Autodesk Inventor part; units mm, degrees
ref_plane "Work Plane1" through (29, 0, 0) normal (0, -1, 0) x (1, 0, 0)
ref_plane "YZ Plane" through (0, 0, 0) normal (1, 0, 0) x (0, 1, 0)
ref_plane "XZ Plane" through (0, 0, 0) normal (0, 1, 0) x (-1, 0, 0)
sketch "Эскиз1" plane through (0, 0, 0) normal (0, 0, 1) x (1, 0, 0)
  line L0 (-1, 0) -> (6, 0)
  line L1 (6, 0) -> (6, 2)
  line L2 (6, 2) -> (2.1, 2)
  line L3 (2.1, 2) -> (1.6705, 2)
  line L4 (1.6705, 2) -> (0, 2)
  line L5 (0, 2) -> (0, 3.5)
  line L6 (0, 3.5) -> (-4, 3.5)
  line L7 (-4, 3.5) -> (-4, 1.7321)
  line L8 (-4, 1.7321) -> (-2, 1.7321)
  line L9 (-2, 1.7321) -> (-1, 0)
  line L10 (-6, 0) -> (8, 0)
  line L11 (0, -0.7) -> (0, 4.2)
  line L12 (2.1, 2) -> (0, 2) construction
  dimension "d1" = 3.9
  dimension "d2" = 0.4295
  dimension "d3" = 4
  dimension "d4" = 2
  dimension "d5" = 60
  dimension "d6" = 4
  dimension "d7" = 4
  dimension "d8" = 3.4641
  dimension "d9" = 7
  dimension "d26" = 6
revolve "Базовый элемент" add sketch "Эскиз1" angle 360 about axis through (-1, 0, 0) along (1, 0, 0)
sketch "Эскиз2" plane through (-4, 0, 0) normal (-1, 0, 0) x (0, 0, 1)
  circle A0 centre (0, 0) radius 1.7321
  line L0 (0, -4.9) -> (0, 4.9)
  line L1 (-4.9, 0) -> (4.9, 0)
  line L2 (1.7321, 0) -> (0.866, -1.5)
  line L3 (0.866, -1.5) -> (-0.866, -1.5)
  line L4 (-0.866, -1.5) -> (-1.7321, 0)
  line L5 (-1.7321, 0) -> (-0.866, 1.5)
  line L6 (-0.866, 1.5) -> (0.866, 1.5)
  line L7 (0.866, 1.5) -> (1.7321, 0)
extrude "Паз" add sketch "Эскиз2" against normal up to next contours L7 A0 | A0 L2 | L6 L0 A0 | A0 L0 L3 | L0 L6 A0 | A0 L3 L0 | L4 A0 | A0 L5
fillet "Сопряжение1" radius 0.4 1 edges at (-4, -3.5, 0)
thread "Резьба"
chamfer "Фаска1" distance 0.4294 distance2 0.4294 1 edges at (6, -2, 0) measured on face at (6, 0.556, 0.0273)
ref_plane "Work Plane1" through (29, 0, 0) normal (0, -1, 0) x (1, 0, 0)
fillet "Fillet2" radius 0.1 1 edges at (0, -2, 0)
equation "\"d1\" = GEL"
equation "\"d3\" = KOH"
equation "\"d4\" = INTI"
equation "\"d6\" = GD"
equation "\"d7\" = BDM"
equation "\"d8\" = 1.1547 * SW"
equation "\"d9\" = KOD"
equation "\"d26\" = NLG"
equation "\"d30\" = R"
equation "\"d17\" = RR"
equation "\"d13\" = GEL"
equation "\"d15\" = -0.5 * SPD + 0.5 * GD"
equation "\"d16\" = GUL"
equation "\"GD\" = NND"
equation "\"NLG\" = 6"
equation "\"GEL\" = 3.9"
equation "\"KOD\" = 7"
equation "\"KOH\" = NND"
equation "\"INTI\" = 2"
equation "\"GAL\" = 0.61345 * PTC"
equation "\"GUL\" = 0.61345 * PTC"
equation "\"BDM\" = NND"
equation "\"SW\" = 3"
equation "\"RR\" = 0.4"
equation "\"SPD\" = NND - 1.2269 * PTC"
equation "\"R\" = 0.1"
equation "\"TOA\" = 30deg"
equation "\"GD1\" = THREADDIA - 1.2269 * PTC"
equation "\"THREADDIA\" = 4"
equation "\"FAWI\" = 45deg"
equation "\"PTC\" = 0.7"
equation "\"NND\" = 4"
equation "\"E0\" = 1.155 * SW"
equation "\"PHH\" = 0"
properties part number "CSN 02 1143 - M4 x 6" material "Сталь, мягкая"
Design review of the part built by this model. Coordinates are the model's own, in mm. A direction names the side the tool comes from. Coordinates: 2 decimals unless noted, no trailing zeros. Order: outer loops, then holes, each group sorted by start corner. A loop starts at its lowest first (then second) coordinate and runs counter-clockwise, first axis right, second up. Notation, with made-up numbers: M -32,28.5 L -27,28.5 A24 ccw -27,55.5 Z; hole C -7,14 d4. An arc over 180 degrees is marked long. Use a Markdown table: item, result.
(1) Draft analysis for pull direction Z (two halves, no side actions). For faces 3 (the cylindrical face through (3, 0, 2)), 4 (the flat face through (0, 2, -2)), 5 (the flat face through (-3, 1.5, 0)), 6 (the flat face through (-2.948, 0.761, 1.293)), state which applies: released by +Z, released by -Z, zero draft, split by the parting line, or undercut.
Worked answers:
| item | result |
|---|---|
| face 3 | split by the parting line |
| face 4 | zero draft |
| face 5 | undercut |
| face 6 | undercut |
(2) Wall thickness on probe 1 along X at (y, z) = (0, 2.5); probe 2 along Z at (x, y) = (3.25, -1); probe 3 along Z at (x, y) = (-2.25, -1): over which ranges is each line inside the solid? List them lowest first.
Worked answers:
| item | result |
|---|---|
| probe 1 | x = -4 to 0 |
| probe 2 | z = -1.73 to 1.73 |
| probe 3 | z = -3.35 to -1.15, 1.15 to 3.35 |
(3) Add section A-A (x = -3). Give the boundary of the cut face in (y, z), then the cut area to 3 significant figures.
Worked answers:
| item | result |
|---|---|
| outline | C 0,0 d7; hole M -1.5,-0.87 L 0,-1.73 L 1.5,-0.87 L 1.5,0.87 L 0,1.73 L -1.5,0.87 Z |
| area | 30.7 mm2 |
(4) For P1, Ø1.5, axis at x = 1, z = 0.5, coming from the -Y side; P2, Ø1.5, axis at x = -1.5, z = -1.5, coming from the -Y side; P3, Ø3, axis at x = 5, y = 1.5, coming from the +Z side, all flat-tipped, find the tip position at first contact; note any pin that passes through.
Worked answers:
| item | result |
|---|---|
| P1 | stops at y = -2 |
| P2 | stops at y = -3.42 |
| P3 | stops at z = 2 |
(5) For faces 1 (the flat face through (-4, -1.3, 1.3)), 2 (the flat face through (-2.948, -0.761, -1.293)), list the 3-axis set-ups (+Z, -Z, +X, -X, +Y, -Y) from which the entire face can be reached by the end or side of a thin tool; tool diameter is ignored.
Worked answers:
| item | result |
|---|---|
| face 1 | +Z, -Z, -X, +Y, -Y |
| face 2 | -X |
(6) Add section B-B (x = 3.75). Give the boundary of the cut face in (y, z), then the cut area to 3 significant figures.
Worked answers:
| item | result |
|---|---|
| outline | C 0,0 d4 |
| area | 12.6 mm2 |
